Part model, mm, in its own coordinate system. A direction names the side the tool comes from. Round coordinates to 2 decimals unless told otherwise and drop trailing zeros. Order: outer loops, then holes, each group sorted by start corner. A loop starts at its lowest first (then second) coordinate and runs counter-clockwise, first axis right, second up. Notation, with made-up numbers: (3, 38.25) - (59, 38.25) arc R36 ccw to (59, 73.25) - close; hole circle Ø7 at (52, 81.25). An arc over 180 degrees is marked (long way). Answer as a JSON object with one key per item and string values.
```python
from build123d import *

# Parameters (mm, degrees)
BOSS_EXTRUDE1_DEPTH     = 100
CUT_EXTRUDE1_DEPTH      = 21
CUT_EXTRUDE1_DEPTH_BACK = 26
SKETCH5_R               = 4
CUT_EXTRUDE2_DEPTH      = 1
CUT_EXTRUDE2_DEPTH_BACK = 82.040159654


with BuildPart() as part:
    # Sketch1 → Boss-Extrude1 (new body)
    with BuildSketch(Plane.XY):
        with BuildLine():
            Line((7.200299815, -5.97393957), (-18.665688958, -77.040159654))
            Line((-18.665688958, -77.040159654), (-32.5, -77.040159654))
            Line((-32.5, -77.040159654), (-7.380922138, -8.02606043))
            ThreePointArc((-7.380922138, -8.02606043), (-7.742543867, -5.279270691), (-10.2, -4))
            Line((-10.2, -4), (-12.5, -4))
            Line((-12.5, -4), (-12.5, 4))
            Line((-12.5, 4), (12.5, 4))
            Line((12.5, 4), (12.5, -4))
            Line((12.5, -4), (10.019377677, -4))
            ThreePointArc((10.019377677, -4), (8.298648368, -4.542543867), (7.200299815, -5.97393957))
        make_face()
    extrude(amount=BOSS_EXTRUDE1_DEPTH)

    # Sketch4 → Cut-Extrude1 (cut, two sides)
    with BuildSketch(Plane.ZY.offset(12.5)) as cut_extrude1_sk:
        with BuildLine():
            ThreePointArc((20, -67.040159654), (12.928932188, -64.111227466), (10, -57.040159654))
            Line((10, -57.040159654), (10, -11))
            Line((10, -11), (90, -11))
            Line((90, -11), (90, -57.040159654))
            ThreePointArc((90, -57.040159654), (87.071067812, -64.111227466), (80, -67.040159654))
            Line((80, -67.040159654), (20, -67.040159654))
        make_face()
        with BuildLine():
            ThreePointArc((100, -57.040159654), (94.142135624, -71.182295278), (80, -77.040159654))
            Line((80, -77.040159654), (100, -77.040159654))
            Line((100, -77.040159654), (100, -57.040159654))
        make_face()
        with BuildLine():
            ThreePointArc((20, -77.040159654), (5.857864376, -71.182295278), (0, -57.040159654))
            Line((0, -57.040159654), (0, -77.040159654))
            Line((0, -77.040159654), (20, -77.040159654))
        make_face()
    extrude(amount=CUT_EXTRUDE1_DEPTH, mode=Mode.SUBTRACT)
    extrude(cut_extrude1_sk.sketch, amount=-CUT_EXTRUDE1_DEPTH_BACK, mode=Mode.SUBTRACT)

    # Sketch5 → Cut-Extrude2 (cut, two sides)
    with BuildSketch(Plane(origin=(0, 4, 0), x_dir=(1, 0, 0), z_dir=(0, 1, 0))) as cut_extrude2_sk:
        with Locations((0, -25)):
            Circle(SKETCH5_R)
        with Locations((0, -75)):
            Circle(SKETCH5_R)
    extrude(amount=CUT_EXTRUDE2_DEPTH, mode=Mode.SUBTRACT)
    extrude(cut_extrude2_sk.sketch, amount=-CUT_EXTRUDE2_DEPTH_BACK, mode=Mode.SUBTRACT)


solid = part.part
```
Item 1: Cut at A-A (z = 75). Write the cut outline in (x, y).
Taken from the geometry:
{"outline": "(-32.5, -77.04) - (-18.67, -77.04) - (-15.03, -67.04) - (-28.86, -67.04) - close; (-12.5, -4) - (-10.2, -4) arc R3 cw to (-7.38, -8.03) - (-8.46, -11) - (-4, -11) - (-4, 4) - (-12.5, 4) - close; (4, -11) - (5.37, -11) - (7.2, -5.97) arc R3 cw to (10.02, -4) - (12.5, -4) - (12.5, 4) - (4, 4) - close"}
Item 2: Cut at C-C (y = -54.5). Write the cut outline in (x, z).
Taken from the geometry:
{"outline": "(-24.3, 0) - (-10.46, 0) - (-10.46, 10) - (-24.3, 10) - close; (-24.3, 90) - (-10.46, 90) - (-10.46, 100) - (-24.3, 100) - close"}
Item 3: Tool access for faces 4 (the flat face through (-29.3, -68.25, 49.77)), 5 (the flat face through (-22, -67.04, 50)), 6 (the cylindrical face through (-0.521, -3.395, 21.034)), 7 (the flat face through (-10, -34, 90)), 8 (the flat face through (11, -4, 49)): list every direction of +Z, -Z, +X, -X, +Y, -Y with a clear straight run to the whole face (end or side of a thin tool).
Taken from the geometry:
{"face 4": "+Z, -Z, -X", "face 5": "+X, -X, +Y", "face 6": "+Y, -Y", "face 7": "+X, -X", "face 8": "+Z, -Z, +X, -Y"}
Item 4: Cut at D-D (z = 44). Write the cut outline in (x, y), plus the area to 3 significant figures.
Taken from the geometry:
{"outline": "(-32.5, -77.04) - (-18.67, -77.04) - (-15.03, -67.04) - (-28.86, -67.04) - close; (-12.5, -4) - (-10.2, -4) arc R3 cw to (-7.38, -8.03) - (-8.46, -11) - (5.37, -11) - (7.2, -5.97) arc R3 cw to (10.02, -4) - (12.5, -4) - (12.5, 4) - (-12.5, 4) - close", "area": "440 mm2"}
Item 5: Cut at B-B (x = 0). Write the cut outline in (y, z), plus the area to 3 significant figures.
Taken from the geometry:
{"outline": "(-25.76, 0) - (4, 0) - (4, 21) - (-11, 21) - (-11, 10) - (-25.76, 10) - close; (-25.76, 90) - (-11, 90) - (-11, 79) - (4, 79) - (4, 100) - (-25.76, 100) - close; (-11, 29) - (4, 29) - (4, 71) - (-11, 71) - close", "area": "1,560 mm2"}
Item 6: Two-plate mould, pull along X, no slides. Class faces 1 (the flat face through (5.944, -9.425, 49.3)), 2 (the cylindrical face through (-0.867, -3.395, 78.905)), 3 (the flat face through (-6, -26, 100)): pulls with the +X half, pulls with the -X half, needs draft (parallel to the pull), parting line crosses it, or undercut.
Taken from the geometry:
{"face 1": "pulls with the +X half", "face 2": "undercut", "face 3": "needs draft"}
Item 7: Probe L1, parallel to Z at x = 0, y = -0.75; L2, parallel to X at y = -0.75, z = 75; L3, parallel to Z at x = -4, y = -33. List the from-to ranges inside material, lowest first. Write a range as from..to.
Taken from the geometry:
{"L1": "0..21, 29..71, 79..100", "L2": "-12.5..-4, 4..12.5", "L3": "0..10, 90..100"}
Item 8: Drop flat-ended pins along their axis: P1, Ø1.5, axis at y = -11.5, z = 54, coming from the +X side; P2, Ø9, axis at x = 0, z = 25, coming from the -Y side; P3, Ø10, axis at y = -9.5, z = 87, coming from the +X side. Give the stop position or say it passes through.
Taken from the geometry:
{"P1": "x = 5.46", "P2": "y = -11", "P3": "x = 8.36"}
